Input: dimensioned drawing with shaded views. Units: mm. Origin: part minimum x, y, z. A direction names the side the tool comes from. Round coordinates to 2 decimals unless told otherwise and drop trailing zeros. Loops run counter-clockwise (first coordinate to the right, second up) from the corner with the lowest first, then second, coordinate; pieces in that order, holes last. Notation, with made-up numbers: (31.25, 78) - (74.25, 78) arc R12 cw to (74.25, 84) - close; hole circle Ø6 at (69.5, 62.25). An arc over 180 degrees is marked (long way). One line per question, with ' | ' between items. Start each with the question number.
1. Cut plane C-C (z = 5.25). Return loops of the section in (x, y), then the cut area to 3 significant figures.
2. Pin query (flat end, axial travel): pin 1 (4 mm diameter, centred on x = 18, z = 5.5, fed in from -Y); pin 2 (1 mm diameter, centred on x = 18, y = 35, fed in from +Z); pin 3 (1.5 mm diameter, centred on x = 8, y = 9.5, fed in from -Z); pin 4 (1.5 mm diameter, centred on x = 7, z = 7, fed in from +Y). Return the tip coordinate at first contact, or that it passes through.
3. Mould query, pull axis X, two halves, no side actions, for the marked faces 3, 4 and 5. Classes: pulls with the +X half, pulls with the -X half, needs draft (parallel to the pull), parting line crosses it, or undercut.
4. Access query for the marked faces 1 and 2. Directions: +Z, -Z, +X, -X, +Y, -Y. A direction counts if a zero-diameter tool reaches every point of the face in a straight line with its end or side. Return the directions, or none.
5. Ray query, line 1 (Z direction, x = 21.25, y = 2); line 2 (Y direction, x = 5.5, z = 6.25); line 3 (Y direction, x = 24, z = 3.5). Return the intervals inside material, ascending.
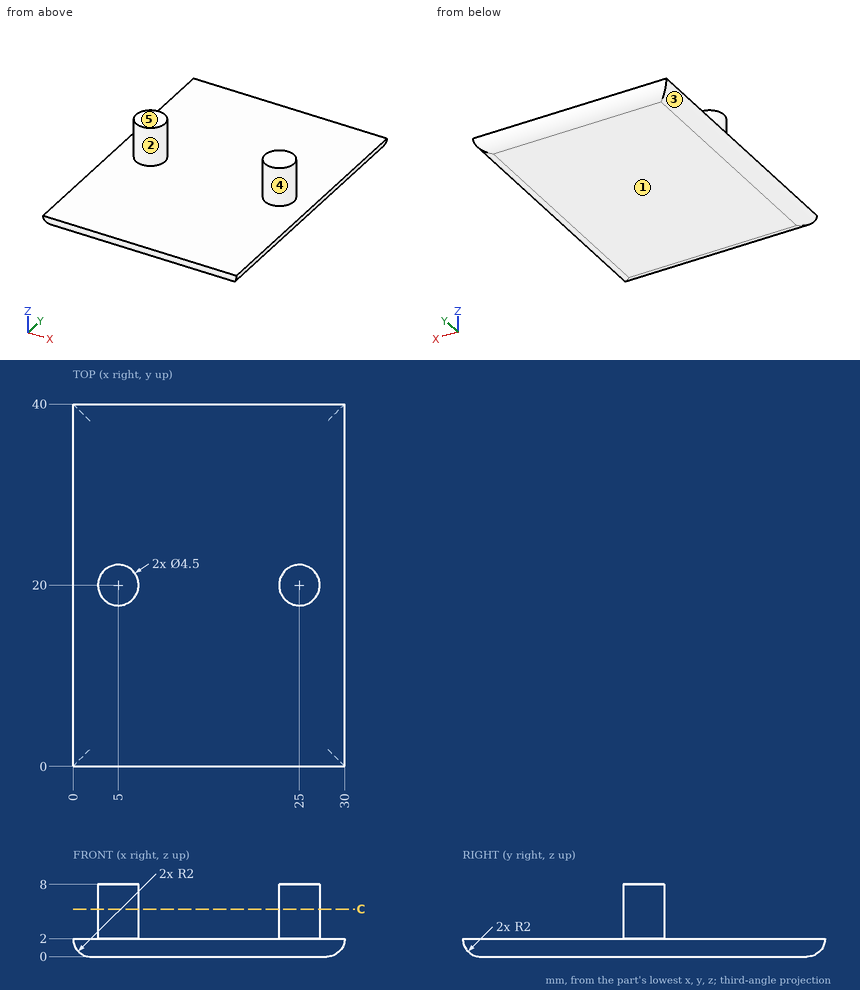
Answers follow:
1) outline: circle Ø4.5 at (5, 20); circle Ø4.5 at (25, 20) | area: 31.8 mm2
2) pin 1: passes through | pin 2: stops at z = 2 | pin 3: stops at z = 0 | pin 4: stops at y = 21.87
3) face 3: pulls with the -X half | face 4: undercut | face 5: needs draft
4) face 1: -Z, +X, -X, +Y, -Y | face 2: +Z
5) line 1: z = 0 to 2 | line 2: y = 17.81 to 22.19 | line 3: y = 17.98 to 22.02
